from build123d import *

# Parameters (mm, degrees)
RESSALTO_EXTRUS_O1_DEPTH = 4


with BuildPart() as part:
    # Esboço1 → Ressalto-extrusão1 (new body)
    with BuildSketch(Plane.XY):
        with BuildLine():
            Line((0, 0), (138, 0))
            ThreePointArc((138, 0), (139.414213562, 0.585786438), (140, 2))
            Line((140, 2), (140, 148.454256327))
            ThreePointArc((140, 148.454256327), (139.414213562, 149.86846989), (138, 150.454256327))
            Line((138, 150.454256327), (9.899407771, 150.454256327))
            Line((9.899407771, 150.454256327), (-41.646512669, 31.110140067))
            ThreePointArc((-41.646512669, 31.110140067), (-41.734695124, 29.77189369), (-40.957602214, 28.678821818))
            Line((-40.957602214, 28.678821818), (0, 0))
        make_face()
    extrude(amount=RESSALTO_EXTRUS_O1_DEPTH)


solid = part.part
CAD build for the part. Positions are in the model's coordinates, mm. Coordinates: 2 decimals unless noted, no trailing zeros. Write each loop counter-clockwise with the first axis right and the second up, starting at its lowest first coordinate (ties: lowest second). Pieces come first, ordered by that corner, then holes. Notation, with made-up numbers: M 85,88 L 99,88 A11 ccw 99,106 Z; hole C 42.25,44.25 d8. An arc over 180 degrees is marked long. Return JSON: item names as keys, results as strings.
Item 1: Slice it at B-B, the plane x = -8. Write the cut outline in (y, z), and give its area (3 significant figures).
Findings below:
{"outline": "M 5.6,0 L 109.01,0 L 109.01,4 L 5.6,4 Z", "area": "414 mm2"}
Item 2: Slice it at C-C, the plane y = 85. Write the cut outline in (x, z).
Findings below:
{"outline": "M -18.37,0 L 140,0 L 140,4 L -18.37,4 Z"}
Item 3: Probe line 1 (X direction, y = 26.5, z = 2.4); line 2 (Y direction, x = -17, z = 3.1); line 3 (Y direction, x = 0.5, z = 1.45). List the from-to ranges inside material, lowest first. Write a range as from..to.
Findings below:
{"line 1": "x = -37.85..140", "line 2": "y = 11.9..88.17", "line 3": "y = 0..128.69"}
Item 4: Slice it at A-A, the plane z = 1.7. Write the cut outline in (x, y).
Findings below:
{"outline": "M -41.65,31.11 A2 ccw -40.96,28.68 L 0,0 L 138,0 A2 ccw 140,2 L 140,148.45 A2 ccw 138,150.45 L 9.9,150.45 Z"}
